Design review of the part built by this model. Coordinates are the model's own, in mm. A direction names the side the tool comes from. Round coordinates to 2 decimals unless told otherwise and drop trailing zeros. Order: outer loops, then holes, each group sorted by start corner. A loop starts at its lowest first (then second) coordinate and runs counter-clockwise, first axis right, second up. Notation, with made-up numbers: M -34.5,28.25 L -10.5,28.25 A18 ccw -10.5,47.25 Z; hole C -15.5,-13 d3. An arc over 180 degrees is marked long. Use a Markdown table: item, result. Add a question column.
(1) For pin 1 (1.8 mm diameter, centred on y = -26.5, z = 2.5, fed in from -X); pin 2 (3 mm diameter, centred on x = 110.5, y = -38, fed in from -Z); pin 3 (10 mm diameter, centred on y = -19, z = 30, fed in from +X); pin 4 (9 mm diameter, centred on x = 122.5, y = -17.5, fed in from -Z), all flat-tipped, find the tip position at first contact; note any pin that passes through.
(2) Machinability: for faces 4 (the face through (121, -29, 6)), 5 (the face through (18.346, -28.857, 13.311)), 6 (the face through (63, -48, 32)), 7 (the face through (5, -29, 6)), which of the approach directions +Z, -Z, +X, -X, +Y, -Y give a long, thin tool a straight path to every point of the face, cutting with its end or side? Answer none if there is none.
(3) Take a section at B-B (z = 4). Write out the cut boundary in (x, y).
(4) The part is to be moulded in two halves that separate along Y. For faces 1 (the face through (63, -30, 27)), 2 (the face through (63, 0, 17)), 3 (the face through (11, -29, 3)), say which applies: released by +Y, released by -Y, zero draft, split by the parting line, or undercut.
(5) To check wall thickness, follow probe 1 along Y at (x, z) = (54, 30.5); probe 2 along X at (y, z) = (-34, 14); probe 3 along Z at (x, y) = (39, -17). State the ranges of each line that lie inside material, in increasing order. Write a range as from..to.
(6) Take a section at D-D (y = -49.5). Write out the cut boundary in (x, z).
(7) Take a section at A-A (y = -29). Write out the cut boundary in (x, z), then the cut area to 3 significant figures.
(8) Take a section at C-C (x = 85.5). Write out the cut boundary in (y, z).
```python
from build123d import *

# Parameters (mm, degrees)
F1_DEPTH = 59
F2_W     = 37
F2_H     = 11
F3_DEPTH = 170
F5_DEPTH = 61.20861
F6_R     = 5


with BuildPart() as f1:
    # F0 (on Front) → F1 (new body)
    with BuildSketch(Plane.XZ):
        with BuildLine():
            Line((11, 6), (11, 0))
            Line((11, 0), (116, 0))
            Line((116, 0), (116, 6))
            Line((116, 6), (127, 6))
            ThreePointArc((127, 6), (119.696249, 28.416488), (98.15559, 38))
            Line((98.15559, 38), (28.84441, 38))
            ThreePointArc((28.84441, 38), (7.303751, 28.416488), (0, 6))
            Line((0, 6), (11, 6))
        make_face()
    extrude(amount=F1_DEPTH)

    # F2 (on Right) → F3 (cut)
    with BuildSketch(Plane.YZ):
        with Locations((-29.5, 32.5)):
            Rectangle(F2_W, F2_H)
    extrude(amount=F3_DEPTH, mode=Mode.SUBTRACT)

    # F4 (on Top) → F5 (cut)
    with BuildSketch(Plane.XY):
        with BuildLine():
            Line((43.84441, -22.5), (24.84441, -22.5))
            ThreePointArc((24.84441, -22.5), (18.34441, -29), (24.84441, -35.5))
            Line((24.84441, -35.5), (43.84441, -35.5))
            ThreePointArc((43.84441, -35.5), (50.34441, -29), (43.84441, -22.5))
        make_face()
        with BuildLine():
            Line((102.15559, -22.5), (83.15559, -22.5))
            ThreePointArc((83.15559, -22.5), (76.65559, -29), (83.15559, -35.5))
            Line((83.15559, -35.5), (102.15559, -35.5))
            ThreePointArc((102.15559, -35.5), (108.65559, -29), (102.15559, -22.5))
        make_face()
    extrude(amount=F5_DEPTH, mode=Mode.SUBTRACT)

    # F6
    f6_edges = [f1.edges().sort_by_distance(p)[0] for p in [
        (7.303751, -59, 28.416488),
        (7.303751, 0, 28.416488),
    ]]
    fillet(f6_edges, radius=F6_R)


solid = f1.part
```
Verdict:
| question | item | result |
|---|---|---|
| 1 | pin 1 | stops at x = 11 |
| 1 | pin 2 | stops at z = 0 |
| 1 | pin 3 | stops at x = 122.34 |
| 1 | pin 4 | stops at z = 6 |
| 2 | face 4 | -Z, +X, +Y, -Y |
| 2 | face 5 | +Z, -Z |
| 2 | face 6 | +Z, +X, -X |
| 2 | face 7 | -Z, -X, +Y, -Y |
| 3 | outline | M 11,-59 L 116,-59 L 116,0 L 11,0 Z; hole M 24.84,-35.5 L 43.84,-35.5 A6.5 ccw 43.84,-22.5 L 24.84,-22.5 A6.5 ccw Z; hole M 83.16,-35.5 L 102.16,-35.5 A6.5 ccw 102.16,-22.5 L 83.16,-22.5 A6.5 ccw Z |
| 4 | face 1 | undercut |
| 4 | face 2 | released by +Y |
| 4 | face 3 | zero draft |
| 5 | probe 1 | y = -59..-48, -11..0 |
| 5 | probe 2 | x = 0.28..20.69, 48..79, 106.31..126.72 |
| 5 | probe 3 | z = 0..27 |
| 6 | outline | M 0,6 L 11,6 L 11,0 L 116,0 L 116,6 L 127,6 A29 ccw 98.16,38 L 28.84,38 A29 ccw Z |
| 7 | outline | M 0,6 L 11,6 L 11,0 L 18.34,0 L 18.34,27 L 6.11,27 A29 ccw Z; M 50.34,0 L 76.66,0 L 76.66,27 L 50.34,27 Z; M 108.66,0 L 116,0 L 116,6 L 127,6 A29 ccw 120.89,27 L 108.66,27 Z |
| 7 | area | 1,500 mm^2 |
| 8 | outline | M -59,0 L -35.5,0 L -35.5,27 L -48,27 L -48,38 L -54,38 A5 ccw -59,33 Z; M -22.5,0 L 0,0 L 0,33 A5 ccw -5,38 L -11,38 L -11,27 L -22.5,27 Z |
